```python
from build123d import *

# Parameters (mm, degrees)
F0_W     = 36
F0_H     = 11
F1_DEPTH = 22.5
F2_DEPTH = 12
F3_DEPTH = 12


with BuildPart() as f1:
    # F0 (on Right) → F1 (new body, symmetric)
    with BuildSketch(Plane.YZ):
        with Locations((18, 5.5)):
            Rectangle(F0_W, F0_H)
        Polygon((0, 22), (0, 11), (36, 11), (36, 40), (25, 40), (25, 30), (14, 30), align=None)
        Polygon((0, 40), (0, 22), (14, 30), (25, 30), (25, 40), align=None)
    extrude(amount=F1_DEPTH, both=True)

    # F0 (on Right) → F2 (cut, symmetric)
    with BuildSketch(Plane.YZ):
        with Locations((18, 5.5)):
            Rectangle(F0_W, F0_H)
    extrude(amount=F2_DEPTH, both=True, mode=Mode.SUBTRACT)

    # F0 (on Right) → F3 (cut, symmetric)
    with BuildSketch(Plane.YZ):
        Polygon((0, 40), (0, 22), (14, 30), (25, 30), (25, 40), align=None)
    extrude(amount=F3_DEPTH, both=True, mode=Mode.SUBTRACT)


solid = f1.part
```
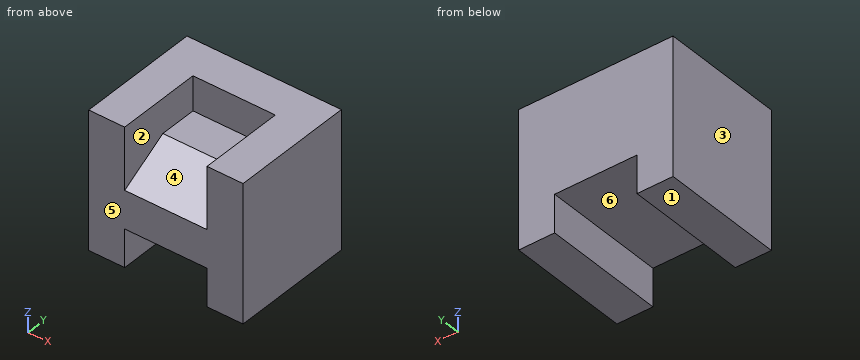
The model under review builds one solid part; all positions refer to its coordinate system, in mm. Face numbers are marked on the shaded views. A direction names the side the tool comes from. Coordinates: 2 decimals unless noted, no trailing zeros. Loops run counter-clockwise (first coordinate to the right, second up) from the corner with the lowest first, then second, coordinate; pieces in that order, holes last. Notation, with made-up numbers: (-30.75, 69) -> (5.25, 69) arc R33 cw to (5.25, 103) -> close; hole circle Ø5 at (27.25, 16). An arc over 180 degrees is marked (long way). Answer as CSV lines item,"result".
Item 1: Take a section at B-B, the plane z = 4. State the section outline as (x, y) points.
Results below:
outline,"(-22.5, 0) -> (-12, 0) -> (-12, 36) -> (-22.5, 36) -> close; (12, 0) -> (22.5, 0) -> (22.5, 36) -> (12, 36) -> close"
Item 2: Machinability: for the marked faces 4, 5 and 6, which of the approach directions +Z, -Z, +X, -X, +Y, -Y give a long, thin tool a straight path to every point of the face, cutting with its end or side? Answer none if there is none.
Results below:
face 4,"+Z, -Y"
face 5,"+Z, -Z, +X, -X, -Y"
face 6,"-Z, +Y, -Y"
Item 3: For L1, parallel to X at y = 28, z = 7.5; L2, parallel to Z at x = 3.5, y = 22; L3, parallel to Y at x = -2.5, z = 37, list the stretches that pass through material, from the lowest coordinate up.
Results below:
L1,"x = -22.5 to -12, 12 to 22.5"
L2,"z = 11 to 30"
L3,"y = 25 to 36"
Item 4: Take a section at A-A, the plane x = 2. State the section outline as (y, z) points.
Results below:
outline,"(0, 11) -> (36, 11) -> (36, 40) -> (25, 40) -> (25, 30) -> (14, 30) -> (0, 22) -> close"
Item 5: Take a section at C-C, the plane y = 17.5. State the section outline as (x, z) points.
Results below:
outline,"(-22.5, 0) -> (-12, 0) -> (-12, 11) -> (12, 11) -> (12, 0) -> (22.5, 0) -> (22.5, 40) -> (12, 40) -> (12, 30) -> (-12, 30) -> (-12, 40) -> (-22.5, 40) -> close"
Item 6: Take a section at D-D, the plane z = 25. State the section outline as (x, y) points.
Results below:
outline,"(-22.5, 0) -> (-12, 0) -> (-12, 5.25) -> (12, 5.25) -> (12, 0) -> (22.5, 0) -> (22.5, 36) -> (-22.5, 36) -> close"
Item 7: Draft analysis for pull direction X (two halves, no side actions). For the marked faces 1, 2 and 3, state which applies: +X half, -X half, draft (parallel to the pull), parting line (faces both ways), or undercut.
Results below:
face 1,"draft"
face 2,"undercut"
face 3,"-X half"
Item 8: Insertion check: pin 1 (9 mm diameter, centred on x = 6, y = 18, fed in from +Z); pin 2 (3 mm diameter, centred on x = -3.5, z = 32.5, fed in from -Y); pin 3 (12 mm diameter, centred on x = 0, y = 16, fed in from -Z); pin 4 (3 mm diameter, centred on x = 15, z = 24.5, fed in from -Y). Each pin has a flat end and moves straight along its axis. Give the tip position at first contact, or say it passes through.
Results below:
pin 1,"stops at z = 30"
pin 2,"stops at y = 25"
pin 3,"stops at z = 11"
pin 4,"stops at y = 0"
